Source: CAD feature listing. Evaluate the final solid. Frame: model axes, mm. A direction names the side the tool comes from. Give positions to 0.01 mm unless a question says otherwise; leave off trailing zeros. Order: outer loops, then holes, each group sorted by start corner. A loop starts at its lowest first (then second) coordinate and runs counter-clockwise, first axis right, second up.
```python
from build123d import *

# Parameters (mm, degrees)
F1_DEPTH     = 25.4
F2_T1_DEPTH  = 78.9172077388
F2_T3_DEPTH  = 19.7233948857
F2_T5_DEPTH  = 65.3813702494
F2_T7_DEPTH  = 81.1736724943
F2_T9_DEPTH  = 51.6358374894
F2_T11_DEPTH = 113.59706738
F2_T14_ANGLE = 90
F2_T19_DEPTH = 93.8736724943
F2_T23_DEPTH = 78.0813702494


# Not quite as in the source:
# - a fillet or chamfer that OpenCascade refuses, or shapes differently, is made with other operations: its cross-section is extruded or revolved along the edge and cut away or added


with BuildPart() as f1:
    # F0 (on Top) → F1 (new body)
    with BuildSketch(Plane.XY):
        with BuildLine():
            Line((-17.2114539891, 42.8890809417), (-36.9348488748, 42.8890809417))
            Line((-36.9348488748, 42.8890809417), (-36.9348488748, 16.6532434523))
            Line((-36.9348488748, 16.6532434523), (-36.9348488748, -23.3281267971))
            ThreePointArc((-36.9348488748, -23.3281267971), (-33.2151049959, -32.3083829181), (-24.2348488748, -36.0281267971))
            Line((-24.2348488748, -36.0281267971), (-17.2114539891, -36.0281267971))
            Line((-17.2114539891, -36.0281267971), (-17.2114539891, 16.6532434523))
            Line((-17.2114539891, 16.6532434523), (51.2622185051, 16.6532434523))
            Line((51.2622185051, 16.6532434523), (51.2622185051, 42.8890809417))
            Line((51.2622185051, 42.8890809417), (-17.2114539891, 42.8890809417))
        make_face()
    extrude(amount=F1_DEPTH)

    # F2: fillet of radius 5.08 on 7 edges, made by hand

    # F2_s2 → F2_t1 (cut)
    with BuildSketch(Plane.XZ.offset(-55.5890809417)):
        with BuildLine():
            add(Edge.make_bspline(
                [(-31.8548488748, 0), (-36.9348488748, 0), (-36.9348488748, 5.08)],
                knots=[0, 0, 0, 1, 1, 1], degree=2, weights=[1, 1, 1]))
            Line((-36.9348488748, 5.08), (-36.9348488748, 0))
            Line((-36.9348488748, 0), (-31.8548488748, 0))
        make_face()
    extrude(amount=F2_T1_DEPTH, mode=Mode.SUBTRACT)

    # F2_s4 → F2_t3 (cut)
    with BuildSketch(Plane.YZ.offset(-24.2348488748)):
        with BuildLine():
            add(Edge.make_bspline(
                [(-36.0281267971, 5.08), (-36.0281267971, 0), (-30.9481267971, 0)],
                knots=[0, 0, 0, 1, 1, 1], degree=2, weights=[1, 1, 1]))
            Line((-30.9481267971, 0), (-36.0281267971, 0))
            Line((-36.0281267971, 0), (-36.0281267971, 5.08))
        make_face()
    extrude(amount=F2_T3_DEPTH, mode=Mode.SUBTRACT)

    # F2_s6 → F2_t5 (cut)
    with BuildSketch(Plane.XZ.offset(-16.6532434523)):
        with BuildLine():
            add(Edge.make_bspline(
                [(-17.2114539891, 5.08), (-17.2114539891, 0), (-22.2914539891, 0)],
                knots=[0, 0, 0, 1, 1, 1], degree=2, weights=[1, 1, 1]))
            Line((-22.2914539891, 0), (-17.2114539891, 0))
            Line((-17.2114539891, 0), (-17.2114539891, 5.08))
        make_face()
    extrude(amount=F2_T5_DEPTH, mode=Mode.SUBTRACT)

    # F2_s8 → F2_t7 (cut)
    with BuildSketch(Plane.YZ.offset(-17.2114539891)):
        with BuildLine():
            add(Edge.make_bspline(
                [(16.6532434523, 5.08), (16.6532434523, 0), (21.7332434523, 0)],
                knots=[0, 0, 0, 1, 1, 1], degree=2, weights=[1, 1, 1]))
            Line((21.7332434523, 0), (16.6532434523, 0))
            Line((16.6532434523, 0), (16.6532434523, 5.08))
        make_face()
    extrude(amount=F2_T7_DEPTH, mode=Mode.SUBTRACT)

    # F2_s10 → F2_t9 (cut)
    with BuildSketch(Plane.XZ.offset(-55.5890809417)):
        with BuildLine():
            add(Edge.make_bspline(
                [(51.2622185051, 5.08), (51.2622185051, 0), (46.1822185051, 0)],
                knots=[0, 0, 0, 1, 1, 1], degree=2, weights=[1, 1, 1]))
            Line((46.1822185051, 0), (51.2622185051, 0))
            Line((51.2622185051, 0), (51.2622185051, 5.08))
        make_face()
    extrude(amount=F2_T9_DEPTH, mode=Mode.SUBTRACT)

    # F2_s12 → F2_t11 (cut)
    with BuildSketch(Plane.YZ.offset(-49.6348488748)):
        with BuildLine():
            add(Edge.make_bspline(
                [(42.8890809417, 5.08), (42.8890809417, 0), (37.8090809417, 0)],
                knots=[0, 0, 0, 1, 1, 1], degree=2, weights=[1, 1, 1]))
            Line((37.8090809417, 0), (42.8890809417, 0))
            Line((42.8890809417, 0), (42.8890809417, 5.08))
        make_face()
    extrude(amount=F2_T11_DEPTH, mode=Mode.SUBTRACT)

    # F2_s13 → F2_t14 (revolve, cut)
    with BuildSketch(Plane.XZ.offset(23.3281267971)):
        with BuildLine():
            add(Edge.make_bspline(
                [(-36.9348488748, 5.08), (-36.9348488748, 0), (-31.8548488748, 0)],
                knots=[0, 0, 0, 1, 1, 1], degree=2, weights=[1, 1, 1]))
            Line((-31.8548488748, 0), (-36.9348488748, 0))
            Line((-36.9348488748, 0), (-36.9348488748, 5.08))
        make_face()
    revolve(axis=Axis((-24.2348488748, -23.3281267971, 0), (0, 0, 1)), revolution_arc=F2_T14_ANGLE, mode=Mode.SUBTRACT)


with BuildPart() as f2_tool17:
    # F2_s18 → F2_t19 (new body)
    with BuildSketch(Plane.YZ.offset(-29.9114539891)):
        with BuildLine():
            add(Edge.make_bspline(
                [(16.6532434523, 5.08), (16.6532434523, 0), (21.7332434523, 0)],
                knots=[0, 0, 0, 1, 1, 1], degree=2, weights=[1, 1, 1]))
            Line((21.7332434523, 0), (16.6532434523, 0))
            Line((16.6532434523, 0), (16.6532434523, 5.08))
        make_face()
    extrude(amount=F2_T19_DEPTH)

    split(bisect_by=Plane.YZ.offset(-17.2114539891), keep=Keep.BOTTOM)


with BuildPart() as f2_tool21:
    # F2_s22 → F2_t23 (new body)
    with BuildSketch(Plane.XZ.offset(48.7281267971)):
        with BuildLine():
            add(Edge.make_bspline(
                [(-17.2114539891, 5.08), (-17.2114539891, 0), (-22.2914539891, 0)],
                knots=[0, 0, 0, 1, 1, 1], degree=2, weights=[1, 1, 1]))
            Line((-22.2914539891, 0), (-17.2114539891, 0))
            Line((-17.2114539891, 0), (-17.2114539891, 5.08))
        make_face()
    extrude(amount=-F2_T23_DEPTH)

    split(bisect_by=Plane.XZ.offset(-16.6532434523), keep=Keep.BOTTOM)


with BuildPart() as f2_tool17_1:
    add(f2_tool17.part)

    # F2_t25: intersect F2_tool21
    add(f2_tool21.part, mode=Mode.INTERSECT)


with BuildPart() as f1_1:
    add(f1.part)

    # F2_t15: cut F2_tool17
    add(f2_tool17_1.part, mode=Mode.SUBTRACT)


solid = f1_1.part
```
1) Reachability of faces 1 (the cylindrical face through (-33.31, -32.21, 15.1)), 2 (the flat face through (17, 16.653, 15)) from +Z, -Z, +X, -X, +Y, -Y: full face, straight path, thin tool, end or side. Return the list, or none.
Report:
face 1: +Z, -Z, -X, -Y
face 2: +Z, -Z, +X, -Y
2) Section query A-A, the plane z = 19. Return the cut outline in (x, y).
Report:
outline: (-36.93, -23.33) arc R12.7 ccw to (-24.23, -36.03) - (-17.21, -36.03) - (-17.21, 16.65) - (51.26, 16.65) - (51.26, 42.89) - (-36.93, 42.89) - close
3) Pin query (flat end, axial travel): pin 1 (10 mm diameter, centred on x = 17, z = 20, fed in from -Y); pin 2 (8 mm diameter, centred on x = 9.5, y = 16, fed in from -Z); pin 3 (1 mm diameter, centred on y = -18.5, z = 3.5, fed in from +X). Return the tip coordinate at first contact, or that it passes through.
Report:
pin 1: stops at y = 16.65
pin 2: stops at z = 0.18
pin 3: stops at x = -17.28
4) Material intervals for L1, parallel to Y at x = 34, z = 16.25; L2, parallel to Y at x = -25, z = 10.5; L3, parallel to X at y = 5.5, z = 9, sorted ascending.
Report:
L1: y = 16.65 to 42.89
L2: y = -36.01 to 42.89
L3: x = -36.93 to -17.21
